Autodesk Inventor part; units mm, degrees
ref_plane "YZ Plane" through (0, 0, 0) normal (1, 0, 0) x (0, 1, 0)
ref_plane "XZ Plane" through (0, 0, 0) normal (0, 1, 0) x (-1, 0, 0)
ref_plane "XY Plane" through (0, 0, 0) normal (0, 0, 1) x (1, 0, 0)
sketch "Sketch1" plane through (0, 0, 0) normal (0, 1, 0) x (-1, 0, 0)
  line L0 (0, 0) -> (50, 0)
  line L1 (50, 0) -> (50, 50)
  line L2 (50, 50) -> (0, 50)
  line L3 (0, 50) -> (0, 0)
  line L4 (50, 50) -> (290, 50)
  line L5 (290, 50) -> (290, 42.5)
  line L6 (290, 42.5) -> (50, 42.5)
  line L7 (50, 42.5) -> (50, 50)
  line L8 (50, 0) -> (290, 0)
  line L9 (290, 0) -> (290, 7.5)
  line L10 (290, 7.5) -> (50, 7.5)
  line L11 (50, 7.5) -> (50, 0)
  dimension "d0" = 50
  dimension "d1" = 50
  dimension "d2" = 240
  dimension "d3" = 7.5
  dimension "d4" = 7.5
extrude "Extrusion1" add sketch "Sketch1" along normal blind 7.5
sketch "Sketch2" plane through (0, 7.5, 0) normal (0, 1, 0) x (1, 0, 0)
  line L0 (0, -50) -> (0, 0)
  point P0 (0, -25)
hole "Hole1" at (0, 7.5, 25) direction (0, -1, 0) diameter 6.35 end through all
sketch "Sketch3" plane through (0, 7.5, 0) normal (0, 1, 0) x (1, 0, 0)
  line L0 (-3.175, -50) -> (-3.175, 0) construction
  line L1 (-3.175, -50) -> (-28.175, -50) construction
  line L2 (-28.175, -50) -> (-28.175, 0) construction
  line L3 (-28.175, 0) -> (-3.175, 0) construction
  point P0 (0, 0)
  point P1 (-7.175, -4)
  point P2 (-24.175, -46)
  dimension "d14" = 25
hole "Hole2" at (-7.175, 7.5, 4) at (-24.175, 7.5, 46) direction (0, -1, 0) diameter 3.3 end through all
sketch "Sketch4" plane through (0, 7.5, 0) normal (0, 1, 0) x (1, 0, 0)
  arc A0 (0, -21.825) -> (0, -28.175) centre (0, -25) ccw construction
  line L0 (-3.175, -25) -> (-28.175, -25) construction
  line L1 (-3.175, -25) -> (21.825, -25) construction
  line L2 (-290, -50) -> (0, -50) construction
  line L3 (-28.175, -50) -> (-28.175, 0) construction
  line L4 (-50, -7.5) -> (-50, -42.5) construction
  line L5 (-50, -42.5) -> (-45, -42.5) construction
  line L6 (-45, -42.5) -> (-45, -32.5) construction
  line L7 (-45, -32.5) -> (-50, -32.5) construction
  line L8 (-50, -32.5) -> (-50, -42.5) construction
  line L9 (-45, -32.5) -> (-40, -32.5)
  line L10 (-40, -32.5) -> (-40, -42.5)
  line L11 (-40, -42.5) -> (-45, -42.5)
  line L12 (-45, -42.5) -> (-45, -32.5)
  point P0 (0, 0)
  dimension "d22" = 25
  dimension "d23" = 180
  dimension "d24" = 5
  dimension "d25" = 10
  dimension "d26" = 5
extrude "Extrusion2" add sketch "Sketch4" along normal blind 17.5
sketch "Sketch5" plane through (0, 7.5, 0) normal (0, 1, 0) x (1, 0, 0)
  line L0 (-85, -7.5) -> (-85, -42.5)
  line L1 (-127.5, -7.5) -> (-127.5, -42.5)
  line L2 (-92.5, -42.5) -> (-92.5, -7.5)
  line L3 (-135, -7.5) -> (-170, -7.5) construction
  line L4 (-170, -7.5) -> (-170, -42.5) construction
  line L5 (-170, -42.5) -> (-135, -42.5) construction
  line L6 (-135, -42.5) -> (-135, -7.5) construction
  line L7 (-177.5, -7.5) -> (-212.5, -7.5) construction
  line L8 (-212.5, -7.5) -> (-212.5, -42.5) construction
  line L9 (-212.5, -42.5) -> (-177.5, -42.5) construction
  line L10 (-177.5, -42.5) -> (-177.5, -7.5) construction
  line L11 (-220, -7.5) -> (-255, -7.5) construction
  line L12 (-255, -7.5) -> (-255, -42.5) construction
  line L13 (-255, -42.5) -> (-220, -42.5) construction
  line L14 (-220, -42.5) -> (-220, -7.5) construction
  line L15 (-85, -7.5) -> (-92.5, -7.5) construction
  line L16 (-92.5, -7.5) -> (-92.5, -42.5) construction
  line L17 (-92.5, -42.5) -> (-85, -42.5) construction
  line L18 (-85, -42.5) -> (-85, -7.5) construction
  line L19 (-127.5, -7.5) -> (-135, -7.5) construction
  line L20 (-135, -7.5) -> (-135, -42.5) construction
  line L21 (-135, -42.5) -> (-127.5, -42.5) construction
  line L22 (-127.5, -42.5) -> (-127.5, -7.5) construction
  line L23 (-170, -7.5) -> (-177.5, -7.5) construction
  line L24 (-177.5, -7.5) -> (-177.5, -42.5) construction
  line L25 (-177.5, -42.5) -> (-170, -42.5) construction
  line L26 (-170, -42.5) -> (-170, -7.5) construction
  line L27 (-212.5, -7.5) -> (-220, -7.5) construction
  line L28 (-220, -7.5) -> (-220, -42.5) construction
  line L29 (-220, -42.5) -> (-212.5, -42.5) construction
  line L30 (-212.5, -42.5) -> (-212.5, -7.5) construction
  line L31 (-220, -7.5) -> (-212.5, -7.5)
  line L32 (-212.5, -7.5) -> (-212.5, -42.5)
  line L33 (-212.5, -42.5) -> (-220, -42.5)
  line L34 (-220, -42.5) -> (-220, -7.5)
  line L35 (-177.5, -7.5) -> (-170, -7.5)
  line L36 (-170, -7.5) -> (-170, -42.5)
  line L37 (-170, -42.5) -> (-177.5, -42.5)
  line L38 (-177.5, -42.5) -> (-177.5, -7.5)
  line L39 (-135, -7.5) -> (-127.5, -7.5)
  line L40 (-127.5, -7.5) -> (-127.5, -42.5)
  line L41 (-127.5, -42.5) -> (-135, -42.5)
  line L42 (-135, -42.5) -> (-135, -7.5)
  line L43 (-92.5, -7.5) -> (-85, -7.5)
  line L44 (-85, -7.5) -> (-85, -42.5)
  line L45 (-85, -42.5) -> (-92.5, -42.5)
  line L46 (-92.5, -42.5) -> (-92.5, -7.5)
  point P0 (0, 0)
  point P1 (-50, -7.5)
  dimension "d30" = 35
  dimension "d31" = 35
  dimension "d32" = 35
  dimension "d33" = 35
  dimension "d34" = 35
  dimension "d35" = 35
extrude "Extrusion3" add sketch "Sketch5" against normal blind 2
sketch "Sketch6" plane through (0, 7.5, 0) normal (0, 1, 0) x (1, 0, 0)
  line L0 (-290, 0) -> (-290, -7.5)
  line L1 (-290, -50) -> (0, -50)
  line L2 (-290, 0) -> (-280, 0)
  line L3 (-280, 0) -> (-280, -50)
  line L4 (-280, -50) -> (-290, -50)
  line L5 (-290, -50) -> (-290, 0)
  point P0 (0, 0)
  dimension "d38" = 10
extrude "Extrusion4" cut sketch "Sketch6" against normal blind 7.5
sketch "Sketch7" plane through (-280, 7.5, 0) normal (-1, 0, 0) x (0, 0, 1)
  point P0 (0, -7.5)
sketch "Sketch8" plane through (-280, 7.5, 0) normal (-1, 0, 0) x (0, 0, 1)
  line L0 (-25, 0) -> (75, 0)
  line L1 (75, 0) -> (75, -7.5)
  line L2 (75, -7.5) -> (-25, -7.5)
  line L3 (-25, -7.5) -> (-25, 0)
  line L4 (-25, 0) -> (75, 0)
  line L5 (75, 0) -> (75, -10)
  line L6 (75, -10) -> (-25, -10)
  line L7 (-25, -10) -> (-25, 0)
  point P0 (0, -7.5)
  dimension "d41" = 100
  dimension "d42" = 10
extrude "Extrusion5" add sketch "Sketch8" along normal blind 7.5
sketch "Sketch9" plane through (-287.5, 7.5, 0) normal (-1, 0, 0) x (0, 0, 1)
  line L0 (75, 0) -> (-25, 0)
  line L1 (-25, -10) -> (75, -10)
  line L2 (-25, 0) -> (-17.5, 0)
  line L3 (-17.5, 0) -> (-17.5, -10)
  line L4 (-17.5, -10) -> (-25, -10)
  line L5 (-25, -10) -> (-25, 0)
  line L6 (75, 0) -> (67.5, 0)
  line L7 (67.5, 0) -> (67.5, -10)
  line L8 (67.5, -10) -> (75, -10)
  line L9 (75, -10) -> (75, 0)
  point P0 (0, -7.5)
  dimension "d45" = 7.5
  dimension "d46" = 7.5
extrude "Extrusion6" add sketch "Sketch9" along normal blind 25 contours L9 L1 L7 L0 | L3 L1 L5 L0
sketch "Sketch10" plane through (-287.5, -2.5, -17.5) normal (0, 0, 1) x (1, 0, 0)
  line L0 (0, 0) -> (-25, 0) construction
  line L1 (0, 0) -> (-3, 0) construction
  line L2 (-3, 0) -> (-6.2, 0)
  line L3 (-6.2, 0) -> (-6.2, 2.1)
  line L4 (-6.2, 2.1) -> (-3, 2.1)
  line L5 (-3, 2.1) -> (-3, 0)
  line L6 (-6.2, 2.1) -> (-11.7, 2.1) construction
  line L7 (-11.7, 2.1) -> (-11.7, 5.4) construction
  point P0 (287.5, 2.5)
  dimension "d49" = 3
  dimension "d50" = 3.2
  dimension "d51" = 2.1
  dimension "d52" = 5.5
  dimension "d53" = 3.3
extrude "Extrusion7" add sketch "Sketch10" along normal blind 92.5
sketch "Sketch11" plane through (-287.5, -2.5, -17.5) normal (0, 0, 1) x (1, 0, 0)
  line L0 (-6.2, 2.1) -> (-3, 2.1) construction
  line L1 (-6.2, 2.1) -> (-11.7, 2.1) construction
  line L2 (-11.7, 2.1) -> (-11.7, 5.4) construction
  circle A0 centre (-11.7, 5.4) radius 2.125
  point P0 (287.5, 2.5)
  dimension "d56" = 5.5
  dimension "d57" = 3.3
  dimension "d58" = 4.25
extrude "Extrusion8" cut sketch "Sketch11" along normal mid plane 241
sketch "Sketch12" plane through (-287.5, -2.5, -17.5) normal (0, 0, 1) x (1, 0, 0)
  circle A0 centre (-11.7, 5.4) radius 2.125 construction
  line L0 (-11.7, 5.4) -> (-11.7, 0.96) construction
  line L1 (-11.7, 0.96) -> (-16.7, 0.96) construction
  line L2 (-6.2, 0) -> (-25, 0)
  line L3 (-16.7, 0.96) -> (-19.2, 0.96)
  line L4 (-19.2, 0.96) -> (-19.2, 0)
  line L5 (-19.2, 0) -> (-16.7, 0)
  line L6 (-16.7, 0) -> (-16.7, 0.96)
  point P0 (287.5, 2.5)
  dimension "d61" = 4.44
  dimension "d62" = 5
  dimension "d63" = 2.5
extrude "Extrusion9" add sketch "Sketch12" along normal blind 91.25
sketch "Sketch13" plane through (-293.7, -0.4, -17.5) normal (0, 1, 0) x (1, 0, 0)
  line L0 (3.2, 0) -> (3.2, -85) construction
  line L1 (3.2, 0) -> (3.2, -30) construction
  line L2 (0, 0) -> (0, -85) construction
  line L3 (3.2, -30) -> (0, -30) construction
  line L4 (0, -30) -> (0, -36.35) construction
  line L5 (0, -36.35) -> (3.2, -36.35) construction
  line L6 (3.2, -36.35) -> (3.2, -30) construction
  line L7 (0, -30) -> (3.2, -30)
  line L8 (3.2, -30) -> (3.2, -36.35)
  line L9 (3.2, -36.35) -> (0, -36.35)
  line L10 (0, -36.35) -> (0, -30)
  point P0 (293.7, -17.5)
  dimension "d66" = 30
  dimension "d67" = 6.35
extrude "Extrusion10" add sketch "Sketch13" along normal blind 3.8
sketch "Sketch14" plane through (0, 7.5, 0) normal (0, 1, 0) x (1, 0, 0)
  line L0 (-287.5, 17.5) -> (-287.5, -67.5)
  line L1 (-287.5, 17.5) -> (-285, 17.5)
  line L2 (-285, 17.5) -> (-285, -67.5)
  line L3 (-285, -67.5) -> (-287.5, -67.5)
  line L4 (-287.5, -67.5) -> (-287.5, 17.5)
  point P0 (0, 0)
  dimension "d70" = 2.5
extrude "Extrusion11" cut sketch "Sketch14" against normal blind 14.55
sketch "Sketch15" plane through (0, 7.5, 0) normal (0, 1, 0) x (1, 0, 0)
  line L0 (-312.5, 17.5) -> (-312.5, 25)
  line L1 (-280, -75) -> (-312.5, -75)
  line L2 (-312.5, 25) -> (-306.6488, 25)
  line L3 (-306.6488, 25) -> (-306.6488, -75)
  line L4 (-306.6488, -75) -> (-312.5, -75)
  line L5 (-312.5, -75) -> (-312.5, 25)
  point P0 (0, 0)
extrude "Extrusion12" cut sketch "Sketch15" against normal blind 14.55
fillet "Fillet1" radius 1 1 edges at (-301.325, 2.9, -17.5)
fillet "Fillet2" radius 1 1 edges at (-301.325, 2.9, 67.5)
fillet "Fillet3" radius 3.25 1 edges at (-280, 2.5, 75)
fillet "Fillet4" radius 3.25 1 edges at (-285, 2.5, 67.5)
fillet "Fillet5" radius 3.25 1 edges at (-280, 2.5, -25)
fillet "Fillet6" radius 3.25 1 edges at (-285, 2.5, -17.5)
sketch "Sketch16" plane through (0, 7.5, 0) normal (0, 1, 0) x (1, 0, 0)
  line L0 (-220, -42.5) -> (-220, -7.5) construction
  line L1 (-220, -42.5) -> (-280, -42.5) construction
  line L2 (-220, -7.5) -> (-255, -7.5) construction
  line L3 (-255, -7.5) -> (-255, -42.5) construction
  line L4 (-255, -42.5) -> (-220, -42.5) construction
  line L5 (-220, -42.5) -> (-220, -7.5) construction
  line L6 (-280, -7.5) -> (-280, 0)
  line L7 (-280, -7.5) -> (-270, -7.5)
  line L8 (-270, -7.5) -> (-270, -42.5)
  line L9 (-270, -42.5) -> (-280, -42.5)
  line L10 (-280, -42.5) -> (-280, -7.5)
  point P0 (0, 0)
  dimension "d81" = 35
  dimension "d82" = 10
extrude "Extrusion13" add sketch "Sketch16" against normal blind 2
sketch "Sketch17" plane through (0, 7.5, 0) normal (0, 1, 0) x (1, 0, 0)
  point P0 (0, 0)
sketch "Sketch18" plane through (0, 7.5, 0) normal (0, 1, 0) x (1, 0, 0)
  line L0 (-270, -7.5) -> (-270, -42.5) construction
  line L1 (-285, -64.25) -> (-285, 14.25) construction
  line L2 (-280, -7.5) -> (-280, 0) construction
  line L3 (-270, -7.5) -> (-280, -7.5) construction
  line L4 (-275, -7.5) -> (-275, -42.5) construction
  line L5 (-50, -42.5) -> (-280, -42.5) construction
  circle A0 centre (-275, -12.5) radius 1.8 construction
  circle A1 centre (-275, -37.5) radius 1.8 construction
  circle A2 centre (-275, -12.5) radius 1.8
  circle A3 centre (-275, -37.5) radius 1.8
  point P0 (0, 0)
  dimension "d85" = 3.6
  dimension "d86" = 3.6
hole "Hole3" at (-275, 7.5, 12.5) at (-275, 7.5, 37.5) direction (0, -1, 0) diameter 3.3 depth 15 tip angle 118
sketch "Sketch19" plane through (0, 7.5, 0) normal (0, 1, 0) x (1, 0, 0)
  circle A0 centre (-275, -12.5) radius 1.65 construction
  line L0 (-275, -12.5) -> (-212.5, -12.5) construction
  line L1 (-212.5, -7.5) -> (-212.5, -42.5) construction
  circle A1 centre (-275, -37.5) radius 1.65 construction
  line L2 (-275, -37.5) -> (-212.5, -37.5) construction
  line L3 (-220, -42.5) -> (-220, -7.5) construction
  line L4 (-220, -12.5) -> (-212.5, -12.5) construction
  line L5 (-216.25, -12.5) -> (-216.25, -37.5) construction
  point P0 (0, 0)
hole "Hole4" at (-216.25, 7.5, 12.5) at (-216.25, 7.5, 37.5) direction (0, -1, 0) diameter 3.3 depth 15 tip angle 118
sketch "Sketch20" plane through (-45, 7.5, 32.5) normal (-1, 0, 0) x (0, 0, 1)
  line L0 (10, 17.5) -> (0, 17.5) construction
  line L1 (5, 17.5) -> (5, -0.1335) construction
  line L2 (10, 0) -> (10, 17.5) construction
  line L3 (10, 12.5) -> (5, 12.5) construction
  circle A0 centre (5, 12.5) radius 3
  point P0 (-32.5, -7.5)
  dimension "d101" = 6
extrude "Extrusion14" cut sketch "Sketch20" against normal blind 20
sketch "Sketch21" plane through (-293.7, -0.4, -17.5) normal (0, 0, 1) x (1, 0, 0)
  circle A0 centre (-5.5, 3.3) radius 2.125 construction
  line L0 (-5.5, 3.3) -> (-5.5, -2.1) construction
  line L1 (0, -2.1) -> (-10.5, -2.1) construction
  line L2 (0, 0) -> (3.2, 0) construction
  line L3 (0, 0) -> (-5.5, 0) construction
  line L4 (-10.5, -1.14) -> (-5.5, -1.14) construction
  line L5 (-10.5, -1.14) -> (-10.5, -2.1) construction
  point P0 (293.7, 0.4)
  dimension "d104" = 3.3
  dimension "d105" = 5.5
  dimension "d106" = 3.2
  dimension "d107" = 4.25
  dimension "d108" = 4.44
  dimension "d109" = 5
  dimension "d110" = 0.96
properties part number "mtv_frame(BrakeInBack)1-13"
Can you work these out from the model? Positions are in its coordinate system, mm. A direction names the side the tool comes from. Give positions to 0.01 mm unless a question says otherwise; leave off trailing zeros. Write each loop counter-clockwise with the first axis right and the second up, starting at its lowest first coordinate (ties: lowest second). Pieces come first, ordered by that corner, then holes. Notation, with made-up numbers: (33, 69) -> (47, 69) arc R19 cw to (47, 84) -> close; hole circle Ø3 at (8, 7). An arc over 180 degrees is marked (long way). Write item = value, one per line.
(1) I'm going to push flat-ended pins straight in: P1, Ø5, axis at x = -36, z = 32, coming from the -Y side; P2, Ø2, axis at x = -76.5, y = 4.5, coming from the -Z side; P3, Ø4.5, axis at x = -7.175, z = 4, coming from the +Y side; P4, Ø6, axis at x = -34.5, y = 21, coming from the -Z side (3 decimals). Where does each tip first touch, or does it pass through?
Worked out:
P1 = 0
P2 = 0
P3 = 7.5
P4 = through
(2) Suppose I cut it at B-B on x = -160. Write out the boundary of the cut face in (y, z), then the cut area to 4 significant figures.
Worked out:
outline = (0, 0) -> (7.5, 0) -> (7.5, 7.5) -> (0, 7.5) -> close; (0, 42.5) -> (7.5, 42.5) -> (7.5, 50) -> (0, 50) -> close
area = 112.5 mm^2
(3) Suppose I cut it at C-C on y = 20. Write out the boundary of the cut face in (x, z).
Worked out:
outline = (-45, 32.5) -> (-40, 32.5) -> (-40, 34.5) -> (-45, 34.5) -> close; (-45, 40.5) -> (-40, 40.5) -> (-40, 42.5) -> (-45, 42.5) -> close
(4) For faces 1 (the face through (-45, 16, 38)), 2 (the face through (-167, 4, 7.5)), 3 (the face through (-290.5, -1, 24)), 4 (the face through (-43, 16, 32.5)), which set-ups out of +Z, -Z, +X, -X, +Y, -Y let a thin tool reach every point of the face, with its end or its side?
Worked out:
face_1 = +Z, -Z, -X, +Y
face_2 = -Y
face_3 = +Y, -Y
face_4 = -Z, +X, -X, +Y
(5) Suppose I cut it at A-A on z = 25. Count the separate pieces of the cut face and the enclosed holes in it, then the cut area to 3 significant figures.
Worked out:
separate_pieces = 8
enclosed_holes = 0
area = 490 mm^2
(6) Thinking about a two-plate mould opening in X: for faces 5 (the face through (-138, 4, 0)), 6 (the face through (-275, 5.5, 25)), 7 (the face through (0, 4, 39)), 8 (the face through (-50, 4, 25)), which applies, released by +X, released by -X, zero draft, split by the parting line, or undercut?
Worked out:
face_5 = zero draft
face_6 = undercut
face_7 = released by +X
face_8 = undercut
(7) I need wall thicknesses on probe 1 along Z at (x, y) = (-275, 6.2); probe 2 along X at (y, z) = (1, 20); probe 3 along X at (y, z) = (2.9, 72) (3 decimals). Which ranges of each line are inside material? Lowest first, please. Write a range as from..to.
Worked out:
probe_1 = 0..10.85, 14.15..35.85, 39.15..50
probe_2 = -285..-280, -50..0
probe_3 = -306.649..-301.325, -297.075..-280.01
